The listing builds one solid part. Answer for the finished solid, in the listing's coordinates (mm). A direction names the side the tool comes from. Round coordinates to 2 decimals unless told otherwise and drop trailing zeros. Write each loop counter-clockwise with the first axis right and the second up, starting at its lowest first coordinate (ties: lowest second). Pieces come first, ordered by that corner, then holes.
(1) A cutting plane is placed at A-A, the plane x = 39. Give the vertices of the cut face in (y, z), and give its area (3 significant figures).
(2) Find the intervals of material crossed by probe 1 along Z at (x, y) = (44, 1.25); probe 2 along X at (y, z) = (1.5, -35); probe 3 along X at (y, z) = (2.5, -34.5), in increasing order.
(3) A cutting plane is placed at B-B, the plane z = -41. Give the vertices of the cut face in (x, y), and give its area (3 significant figures).
(4) A cutting plane is placed at D-D, the plane x = 47. Give the vertices of the cut face in (y, z), and give its area (3 significant figures).
(5) A cutting plane is placed at C-C, the plane z = -28. Give the vertices of the cut face in (x, y), and give its area (3 significant figures).
(6) Each of these flat-tipped pins is pushed along its axis until it touches: pin 1 Ø3 at (x, z) = (26.44, -34.28) entering from +Y; pin 2 Ø2 at (y, z) = (2, -12) entering from +X; pin 3 Ø2 at (y, z) = (2.5, -12.5) entering from -X; pin 4 Ø3 at (x, y) = (18.5, 6) entering from -Z. Where does it stop, or does it pass through?
(7) The mould has two halves that part along X. Classify faces 6 (the face through (43, 3, 0.496)), 7 (the face through (42, 7, -10)), 8 (the face through (74.427, 3.451, -6.312)): +X half, -X half, draft (parallel to the pull), parting line (faces both ways), or undercut.
(8) For faces 1 (the face through (11.14, 3.45, -6.68)), 2 (the face through (43, 4, -38.4)), 3 (the face through (24.848, 3.451, -51.074)), 4 (the face through (42, 0, -10)), 5 (the face through (60.848, 3.451, -51.026)), determine the directions among +Z, -Z, +X, -X, +Y, -Y from which every point of the face is accessible in a straight line to the end or side of a thin tool.
from build123d import *

# Parameters (mm, degrees)
BOSS_EXTRUDE3_DEPTH = 7
SKETCH2_R           = 1.6
SKETCH2_W           = 26.3
SKETCH2_H           = 8.2
CUT_EXTRUDE1_DEPTH  = 8


with BuildPart() as part:
    # Sketch1 → Boss-Extrude3 (new body)
    with BuildSketch(Plane(origin=(0, 0, 0), x_dir=(1, 0, 0), z_dir=(0, 1, 0))):
        Polygon((29.1090159, -7.44261314), (29.140104813, -0.496460718), (42.890104813, -0.496460718), (56.640104813, -0.496460718), (56.671193726, -7.44261314), (61.001320745, -9.94261314), (67.032409659, -6.496460718), (82.032409659, 19.484301396), (82.001320745, 26.430453819), (77.671193726, 28.930453819), (71.640104813, 25.484301396), (64.765104813, 37.392150698), (57.890104813, 49.3), (63.890104813, 52.8), (63.890104813, 57.8), (57.890104813, 61.3), (27.890104813, 61.3), (21.890104813, 57.8), (21.890104813, 52.8), (27.890104813, 49.3), (21.015104813, 37.392150698), (14.140104813, 25.484301396), (8.1090159, 28.930453819), (3.778888881, 26.430453819), (3.747799968, 19.484301396), (18.747799968, -6.496460718), (24.778888881, -9.94261314), align=None)
    extrude(amount=BOSS_EXTRUDE3_DEPTH)

    # Sketch2 → Cut-Extrude1 (cut, through all)
    with BuildSketch(Plane(origin=(0, 7, 0), x_dir=(1, 0, 0), z_dir=(0, 1, 0))):
        with Locations((59.342544079, 34.284301396)):
            Circle(SKETCH2_R)
        with Locations((59.342544079, 14.984301396)):
            Circle(SKETCH2_R)
        with Locations((26.437665547, 14.984301396)):
            Circle(SKETCH2_R)
        with Locations((26.437665547, 34.284301396)):
            Circle(SKETCH2_R)
        with BuildLine():
            Line((34.740104813, 11.003539282), (51.040104813, 11.003539282))
            Line((51.040104813, 11.003539282), (51.040104813, 15.284876488))
            ThreePointArc((51.040104813, 15.284876488), (42.890104813, 37.262613559), (34.740104813, 15.284876488))
            Line((34.740104813, 15.284876488), (34.740104813, 11.003539282))
        make_face()
        with Locations((42.890104813, 42.5)):
            Rectangle(SKETCH2_W, SKETCH2_H)
    extrude(amount=-CUT_EXTRUDE1_DEPTH, mode=Mode.SUBTRACT)


solid = part.part
Solutions:
1. outline: (0, -61.3) - (7, -61.3) - (7, -46.6) - (0, -46.6) - close; (0, -38.4) - (7, -38.4) - (7, -36.64) - (0, -36.64) - close; (0, -11) - (7, -11) - (7, 0.5) - (0, 0.5) - close
1. area: 196 mm2
2. probe 1: z = -61.3 to -46.6, -38.4 to -37.21, -11 to 0.5
2. probe 2: x = 19.63 to 25.01, 27.87 to 35.72, 50.06 to 57.91, 60.77 to 66.15
2. probe 3: x = 19.35 to 24.85, 28.02 to 35.05, 50.73 to 57.76, 60.93 to 66.43
3. outline: (23.1, 0) - (29.74, 0) - (29.74, 7) - (23.1, 7) - close; (56.04, 0) - (62.68, 0) - (62.68, 7) - (56.04, 7) - close
3. area: 93.0 mm2
4. outline: (0, -61.3) - (7, -61.3) - (7, -46.6) - (0, -46.6) - close; (0, -38.4) - (7, -38.4) - (7, -36.57) - (0, -36.57) - close; (0, -11) - (7, -11) - (7, 0.5) - (0, 0.5) - close
4. area: 196 mm2
5. outline: (6.5, 0) - (9.74, 0) - (9.74, 7) - (6.5, 7) - close; (15.59, 0) - (30.82, 0) - (30.82, 7) - (15.59, 7) - close; (54.96, 0) - (70.19, 0) - (70.19, 7) - (54.96, 7) - close; (76.04, 0) - (79.28, 0) - (79.28, 7) - (76.04, 7) - close
5. area: 258 mm2
6. pin 1: passes through
6. pin 2: stops at x = 78.29
6. pin 3: stops at x = 7.2
6. pin 4: stops at z = -35.63
7. face 6: undercut
7. face 7: draft
7. face 8: +X half
8. face 1: +Z, -X, +Y, -Y
8. face 2: +Y, -Y
8. face 3: -X, +Y, -Y
8. face 4: +Z, -Z, +X, -X, -Y
8. face 5: +X, +Y, -Y
